For this review, take the finished solid that the model builds, in its own axes (mm). Face numbers are marked on the shaded views. A direction names the side the tool comes from. Give positions to 0.01 mm unless a question says otherwise; leave off trailing zeros. Loops run counter-clockwise (first coordinate to the right, second up) from the corner with the lowest first, then second, coordinate; pieces in that order, holes last.
```python
from build123d import *

# Parameters (mm, degrees)
SKETCH1_W           = 12.7
SKETCH1_H           = 9.525
BOSS_EXTRUDE1_DEPTH = 2.54
FILLET1_R           = 0.635
SHELL1_START        = 0.635
SHELL1_OUTLINE_W    = 1.905
SHELL1_OUTLINE_H    = 8.255
SHELL1_DEPTH        = 11.43
SKETCH2_R           = 2.54
BOSS_EXTRUDE2_DEPTH = 1.905


# Read off the part's stored shape, not the designer's step: Shell1
with BuildPart() as part:
    # Sketch1 → Boss-Extrude1 (new body)
    with BuildSketch(Plane(origin=(0, 0, 0), x_dir=(1, 0, 0), z_dir=(0, 1, 0))):
        with Locations((6.35, 4.7625)):
            Rectangle(SKETCH1_W, SKETCH1_H)
    extrude(amount=BOSS_EXTRUDE1_DEPTH)

    # Fillet1
    fillet1_edges = [part.edges().sort_by_distance(p)[0] for p in [
        (0, 1.27, -9.525),
        (12.7, 1.27, -9.525),
        (12.7, 1.27, 0),
        (0, 1.27, 0),
    ]]
    fillet(fillet1_edges, radius=FILLET1_R)

    # Shell1 outline → Shell1 (cut)
    with BuildSketch(Plane.YZ.offset(SHELL1_START)):
        with Locations((0.9525, -4.7625)):
            Rectangle(SHELL1_OUTLINE_W, SHELL1_OUTLINE_H)
    extrude(amount=SHELL1_DEPTH, mode=Mode.SUBTRACT)

    # Sketch2 → Boss-Extrude2 (add)
    with BuildSketch(Plane(origin=(0, 1.905, 0), x_dir=(-1, 0, 0), z_dir=(0, -1, 0))):
        with Locations(Location((-6.35, 4.7625, 0), (0, 0, 270))):
            Circle(SKETCH2_R)
    extrude(amount=BOSS_EXTRUDE2_DEPTH)


solid = part.part
```
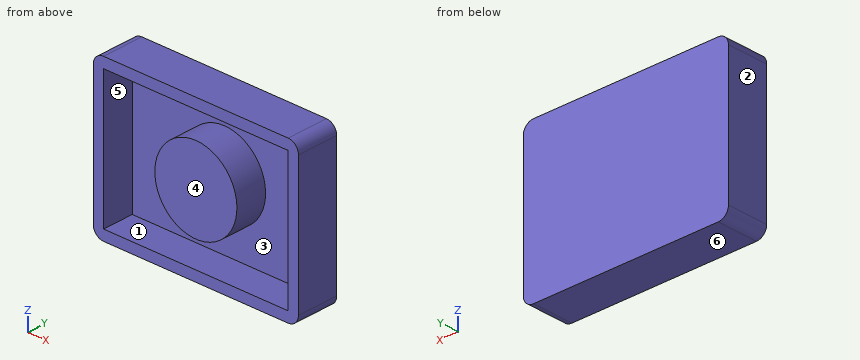
Item 1: Tool access review of the marked faces 1 and 2: name each direction out of +Z, -Z, +X, -X, +Y, -Y from which nothing blocks a thin tool from reaching the whole face with its end or side.
Answer:
face 1: -Y
face 2: +Z, -Z, -X, +Y, -Y
Item 2: Take a section at D-D on z = -5.25. Give the boundary of the cut face in (x, y) (3 decimals), and give its area (3 significant figures).
Answer:
outline: (0, 0) - (0.635, 0) - (0.635, 1.905) - (3.857, 1.905) - (3.857, 0) - (8.843, 0) - (8.843, 1.905) - (12.065, 1.905) - (12.065, 0) - (12.7, 0) - (12.7, 2.54) - (0, 2.54) - close
area: 20.0 mm2
Item 3: Take a section at C-C on z = -1.5. Give the boundary of the cut face in (x, y) (3 decimals), and give its area (3 significant figures).
Answer:
outline: (0, 0) - (0.635, 0) - (0.635, 1.905) - (12.065, 1.905) - (12.065, 0) - (12.7, 0) - (12.7, 2.54) - (0, 2.54) - close
area: 10.5 mm2
Item 4: For L1, parallel to Z at x = 9.75, y = 1.75 (3 decimals); L2, parallel to X at y = 0.75, z = -6.75 (3 decimals); L3, parallel to X at y = 1.35, z = -4.5 (3 decimals), list the stretches that pass through material, from the lowest coordinate up.
Answer:
L1: z = -9.525 to -8.89, -0.635 to 0
L2: x = 0 to 0.635, 4.768 to 7.932, 12.065 to 12.7
L3: x = 0 to 0.635, 3.824 to 8.876, 12.065 to 12.7
Item 5: Clearance check with a flat-ended pin moving along its axis: pin 1 Ø3 at (x, z) = (9, -6) entering from -Y. State where the tip first meets the part, or that it passes through.
Answer:
pin 1: stops at y = 0
Item 6: Take a section at A-A on y = 0.75. State how many separate pieces and enclosed holes the cut face has, and give its area (3 significant figures).
Answer:
separate pieces: 2
enclosed holes: 1
area: 46.5 mm2
Item 7: The part is to be moulded in two halves that separate along Z. For the marked faces 3, 4, 5 and 6, say which applies: released by +Z, released by -Z, zero draft, split by the parting line, or undercut.
Answer:
face 3: undercut
face 4: zero draft
face 5: undercut
face 6: released by -Z
Item 8: Take a section at B-B on x = 6.35. Give the boundary of the cut face in (y, z) (1 decimal).
Answer:
outline: (0, -9.5) - (2.5, -9.5) - (2.5, 0) - (0, 0) - (0, -0.6) - (1.9, -0.6) - (1.9, -2.2) - (0, -2.2) - (0, -7.3) - (1.9, -7.3) - (1.9, -8.9) - (0, -8.9) - close
